```python
from build123d import *

# Parameters (mm, degrees)
F0_W     = 153.19502
F0_H     = 119.012598
F0_R     = 1.5875
F1_DEPTH = 3.175
F2_DEPTH = 3.175


with BuildPart() as f1:
    # F0 (on Top) → F1 (new body)
    with BuildSketch(Plane.XY):
        Polygon((76.59751, 50.750098), (76.59751, -68.2625), (-76.59751, -68.2625), (-76.59751, 50.750098), (-81.36001, 50.750098), (-81.36001, -73.025), (81.36001, -73.025), (81.36001, 50.750098), align=None)
        with Locations((0, -8.756201)):
            Rectangle(F0_W, F0_H)
        with Locations((-34.163, -31.75)):
            Circle(F0_R, mode=Mode.SUBTRACT)
        with Locations((34.163, -31.75)):
            Circle(F0_R, mode=Mode.SUBTRACT)
        with Locations((-28.575, 0)):
            Circle(F0_R, mode=Mode.SUBTRACT)
        with Locations((-34.163, 31.75)):
            Circle(F0_R, mode=Mode.SUBTRACT)
        with Locations((28.575, 0)):
            Circle(F0_R, mode=Mode.SUBTRACT)
        with Locations((34.163, 31.75)):
            Circle(F0_R, mode=Mode.SUBTRACT)
    extrude(amount=F1_DEPTH)

    # F0 (on Top) → F2 (join)
    with BuildSketch(Plane.XY):
        Polygon((76.59751, 50.750098), (76.59751, -68.2625), (-76.59751, -68.2625), (-76.59751, 50.750098), (-81.36001, 50.750098), (-81.36001, -73.025), (81.36001, -73.025), (81.36001, 50.750098), align=None)
    extrude(amount=-F2_DEPTH)


solid = f1.part
```
CAD build for the part. Positions are in the model's coordinates, mm. A direction names the side the tool comes from. Give positions to 0.01 mm unless a question says otherwise; leave off trailing zeros. Write each loop counter-clockwise with the first axis right and the second up, starting at its lowest first coordinate (ties: lowest second). Pieces come first, ordered by that corner, then holes. Notation, with made-up numbers: M 11.5,44.25 L 22.5,44.25 A26 cw 22.5,75.25 Z; hole C 60.25,43 d6. An arc over 180 degrees is marked long. Return JSON: item names as keys, results as strings. Group by question number.
(1) Band-saw the part on A-A (z = -1.25). Give the cut face in (x, y) (1 decimal).
(2) Mould opens along X. For faces 1 (the face through (-1, -10, 3.175)), 2 (the face through (35.677, -31.273, 1.565)), 3 (the face through (81.36, -12, 0)), 4 (the face through (-32.65, -31.27, 1.57)) say: pulls with the +X half, pulls with the -X half, needs draft (parallel to the pull), parting line crosses it, or undercut.
(3) Flat gauge pins, fed straight in: pin 1 Ø2.5 at (x, y) = (-34.163, 31.75) entering from +Z; pin 2 Ø2.5 at (x, z) = (20, -1.5) entering from +Y; pin 3 Ø5 at (x, y) = (-4, -42.5) entering from -Z. Where does each tip first touch, or does it go through?
(4) Drill centre lines: L1, parallel to X at y = -34, z = -3; L2, parallel to Y at x = 35, z = 3 (3 decimals); L3, parallel to X at y = -32.5, z = 0.75. Where is each one in solid material? Low to high. Write a range as [from, to].
(5) Band-saw the part on B-B (y = -20). Give the cut face in (x, z) (1 decimal).
(6) 3-axis set-ups, long thin cutter, end or side, ignore diameter. For faces 5 (the face through (-76.598, -10, -2)), 6 (the face through (-32.65, 32.23, 1.57)): which of +Z, -Z, +X, -X, +Y, -Y reach the whole face in a straight line?
(7) Band-saw the part on C-C (x = 65.5). Give the cut face in (y, z) (1 decimal).
Entries:
{
 "1": {"outline": "M -81.4,-73 L 81.4,-73 L 81.4,50.8 L 76.6,50.8 L 76.6,-68.3 L -76.6,-68.3 L -76.6,50.8 L -81.4,50.8 Z"},
 "2": {"face 1": "needs draft", "face 2": "undercut", "face 3": "pulls with the +X half", "face 4": "undercut"},
 "3": {"pin 1": "passes through", "pin 2": "stops at y = -68.26", "pin 3": "stops at z = 0"},
 "4": {"L1": "x = [-81.36, -76.6], [76.6, 81.36]", "L2": "y = [-73.025, -33.099], [-30.401, 30.401], [33.099, 50.75]", "L3": "x = [-81.36, -35.56], [-32.76, 32.76], [35.56, 81.36]"},
 "5": {"outline": "M -81.4,-3.2 L -76.6,-3.2 L -76.6,0 L 76.6,0 L 76.6,-3.2 L 81.4,-3.2 L 81.4,3.2 L -81.4,3.2 Z"},
 "6": {"face 5": "-Z, +Y", "face 6": "+Z, -Z"},
 "7": {"outline": "M -73,-3.2 L -68.3,-3.2 L -68.3,0 L 50.8,0 L 50.8,3.2 L -73,3.2 Z"}
}
